from build123d import *

# Parameters (mm, degrees)
EXTRUDE_THIN2_DEPTH     = 165.4
SKETCH11_W              = 166
SKETCH11_H              = 4
BOSS_EXTRUDE3_DEPTH     = 2.6416
CUT_EXTRUDE6_DEPTH      = 270.69086006
CUT_EXTRUDE6_DEPTH_BACK = 270.69086006
SKETCH13_W              = 110.495011338
SKETCH13_H              = 5
CUT_EXTRUDE7_DEPTH      = 273.127102656
SKETCH19_W              = 4
SKETCH19_H              = 155.4
CUT_EXTRUDE9_DEPTH      = 10
SKETCH20_W              = 4
SKETCH20_H              = 155.4
CUT_EXTRUDE10_DEPTH     = 10
SKETCH21_W              = 6
SKETCH21_H              = 86.697
BOSS_EXTRUDE4_DEPTH     = 110
CUT_EXTRUDE11_DEPTH     = 4
SKETCH23_W              = 166
SKETCH23_H              = 4
BOSS_EXTRUDE5_DEPTH     = 2.6416
SKETCH24_W              = 4.14
SKETCH24_H              = 4
BOSS_EXTRUDE6_DEPTH     = 49.64
SKETCH25_W              = 4.14
SKETCH25_H              = 4
BOSS_EXTRUDE7_DEPTH     = 49.64
SKETCH26_W              = 4.14
SKETCH26_H              = 4
BOSS_EXTRUDE8_DEPTH     = 49.64
SKETCH27_W              = 4.14
SKETCH27_H              = 4
BOSS_EXTRUDE9_DEPTH     = 49.64


with BuildPart() as part:
    # Sketch2 → Extrude-Thin2 (new body)
    with BuildSketch(Plane.XY):
        Polygon((0, 120), (0, 0), (186, 0), (186, 120), (176, 120), (176, 10), (10, 10), (10, 120), align=None)
    extrude(amount=EXTRUDE_THIN2_DEPTH)

    # Sketch11 → Boss-Extrude3 (add)
    with BuildSketch(Plane(origin=(0, 10, 0), x_dir=(1, 0, 0), z_dir=(0, 1, 0))):
        with Locations((93, -34.703)):
            Rectangle(SKETCH11_W, SKETCH11_H)
    extrude(amount=BOSS_EXTRUDE3_DEPTH)

    # Sketch13 → Cut-Extrude6 (cut, two sides: drawn at the far end of the back side and taken through both)
    with BuildSketch(Plane(origin=(10, 0, 0), x_dir=(0, 0, -1), z_dir=(1, 0, 0)).offset(-CUT_EXTRUDE6_DEPTH_BACK)):
        with Locations((-103.947505669, 89.551599899)):
            Rectangle(SKETCH13_W, SKETCH13_H)
    extrude(amount=CUT_EXTRUDE6_DEPTH + CUT_EXTRUDE6_DEPTH_BACK, mode=Mode.SUBTRACT)

    # Sketch14 → Cut-Extrude7 (cut, through all)
    with BuildSketch(Plane(origin=(0, 10, 0), x_dir=(1, 0, 0), z_dir=(0, 1, 0))):
        with BuildLine():
            Line((176, -165.4), (10, -165.4))
            ThreePointArc((10, -165.4), (93, -135.4), (176, -165.4))
        make_face()
    extrude(amount=-CUT_EXTRUDE7_DEPTH, mode=Mode.SUBTRACT)

    # Sketch19 → Cut-Extrude9 (cut)
    with BuildSketch(Plane(origin=(0, 120, 0), x_dir=(1, 0, 0), z_dir=(0, 1, 0))):
        with Locations((5, -82.7)):
            Rectangle(SKETCH19_W, SKETCH19_H)
    extrude(amount=-CUT_EXTRUDE9_DEPTH, mode=Mode.SUBTRACT)

    # Sketch20 → Cut-Extrude10 (cut)
    with BuildSketch(Plane(origin=(0, 120, 0), x_dir=(1, 0, 0), z_dir=(0, 1, 0))):
        with Locations((181, -82.7)):
            Rectangle(SKETCH20_W, SKETCH20_H)
    extrude(amount=-CUT_EXTRUDE10_DEPTH, mode=Mode.SUBTRACT)

    # Sketch21 → Boss-Extrude4 (add, through all)
    with BuildSketch(Plane(origin=(0, 10, 0), x_dir=(1, 0, 0), z_dir=(0, 1, 0))):
        with Locations((93, -82.0515)):
            Rectangle(SKETCH21_W, SKETCH21_H)
    extrude(amount=BOSS_EXTRUDE4_DEPTH)

    # Sketch22 → Cut-Extrude11 (cut)
    with BuildSketch(Plane(origin=(0, 10, 0), x_dir=(1, 0, 0), z_dir=(0, 1, 0))):
        Polygon((36, -48.703), (36, -148.583194008), (42, -145.837577441), (42, -48.703), align=None)
        Polygon((144, -145.837577441), (150, -148.583194008), (150, -48.703), (144, -48.703), align=None)
    extrude(amount=-CUT_EXTRUDE11_DEPTH, mode=Mode.SUBTRACT)

    # Sketch23 → Boss-Extrude5 (add)
    with BuildSketch(Plane(origin=(0, 10, 0), x_dir=(1, 0, 0), z_dir=(0, 1, 0))):
        with Locations((93, -27.263)):
            Rectangle(SKETCH23_W, SKETCH23_H)
    extrude(amount=BOSS_EXTRUDE5_DEPTH)

    # Sketch24 → Boss-Extrude6 (add)
    with BuildSketch(Plane(origin=(0, 12.6416, 0), x_dir=(1, 0, 0), z_dir=(0, 1, 0))):
        with Locations((12.07, -27.263)):
            Rectangle(SKETCH24_W, SKETCH24_H)
    extrude(amount=BOSS_EXTRUDE6_DEPTH)

    # Sketch25 → Boss-Extrude7 (add)
    with BuildSketch(Plane(origin=(0, 12.6416, 0), x_dir=(1, 0, 0), z_dir=(0, 1, 0))):
        with Locations((173.93, -27.263)):
            Rectangle(SKETCH25_W, SKETCH25_H)
    extrude(amount=BOSS_EXTRUDE7_DEPTH)

    # Sketch26 → Boss-Extrude8 (add)
    with BuildSketch(Plane(origin=(0, 12.6416, 0), x_dir=(1, 0, 0), z_dir=(0, 1, 0))):
        with Locations((12.07, -34.703)):
            Rectangle(SKETCH26_W, SKETCH26_H)
    extrude(amount=BOSS_EXTRUDE8_DEPTH)

    # Sketch27 → Boss-Extrude9 (add)
    with BuildSketch(Plane(origin=(0, 12.6416, 0), x_dir=(1, 0, 0), z_dir=(0, 1, 0))):
        with Locations((173.93, -34.703)):
            Rectangle(SKETCH27_W, SKETCH27_H)
    extrude(amount=BOSS_EXTRUDE9_DEPTH)


solid = part.part
Check sheet for the modelled part. Datum: model origin and axes. Units: mm. A direction names the side the tool comes from. Give positions to 0.01 mm unless a question says otherwise; leave off trailing zeros. Write each loop counter-clockwise with the first axis right and the second up, starting at its lowest first coordinate (ties: lowest second). Pieces come first, ordered by that corner, then holes. Notation, with made-up numbers: (30, -4) -> (51, -4) arc R23 ccw to (51, 8) -> close; hole circle Ø8 at (-33, 22.25). An arc over 180 degrees is marked (long way). One line per item, written item: value. Start each with the question number.
Item 1: Tool access check on faces 1 (the flat face through (5, 90, 48.7)), 2 (the flat face through (39, 6, 98)), 3 (the flat face through (179, 115, 84)), 4 (the flat face through (93, 11, 25.263)), 5 (the flat face through (181, 87.052, 105)). Record the directions out of +Z, -Z, +X, -X, +Y, -Y that give a thin tool (end or side, any length) a straight path to the whole face; none if there is none.
Item 2: Draft check along Z on faces 6 (the flat face through (76, 10, 86)), 7 (the flat face through (7, 115, 84)), 8 (the flat face through (5, 61, 165.4)). Enter one of: +Z half, -Z half, draft (parallel to the pull), parting line (faces both ways), or undercut.
Item 3: Section check D-D on y = 49. Record the cut outline in (x, z).
Item 4: Section check A-A on y = 75. Record the cut outline in (x, z), then the cut area to 3 significant figures.
Item 5: Material ranges on probe 1 along X at (y, z) = (16.5, 46.5); probe 2 along X at (y, z) = (71.5, 9.5); probe 3 along X at (y, z) = (50, 27), recorded low to high. Write a range as from..to.
Item 6: Section check C-C on x = 147. Record the cut outline in (y, z), then the cut area to 3 significant figures.
Item 7: Section check B-B on z = 10.5. Record the cut outline in (x, y), then the cut area to 3 significant figures.
Item 8: Gauge pin test, flat ends, axial feed: pin 1 (4.5 mm diameter, centred on x = 173.5, z = 34.5, fed in from +Y); pin 2 (3 mm diameter, centred on x = 44, z = 144.5, fed in from +Y); pin 3 (10 mm diameter, centred on x = 115.5, y = 16, fed in from +Z). Record the tip position at first contact, or that the pin passes through.
Results list:
1. face 1: -X
1. face 2: +Z, +Y
1. face 3: +Y
1. face 4: -Z, +Y
1. face 5: +X
2. face 6: draft
2. face 7: undercut
2. face 8: +Z half
3. outline: (0, 0) -> (10, 0) -> (10, 25.26) -> (14.14, 25.26) -> (14.14, 29.26) -> (10, 29.26) -> (10, 32.7) -> (14.14, 32.7) -> (14.14, 36.7) -> (10, 36.7) -> (10, 165.4) -> (0, 165.4) -> close; (90, 38.7) -> (96, 38.7) -> (96, 125.4) -> (90, 125.4) -> close; (171.86, 25.26) -> (176, 25.26) -> (176, 0) -> (186, 0) -> (186, 165.4) -> (176, 165.4) -> (176, 36.7) -> (171.86, 36.7) -> (171.86, 32.7) -> (176, 32.7) -> (176, 29.26) -> (171.86, 29.26) -> close
4. outline: (0, 0) -> (10, 0) -> (10, 165.4) -> (0, 165.4) -> close; (90, 38.7) -> (96, 38.7) -> (96, 125.4) -> (90, 125.4) -> close; (176, 0) -> (186, 0) -> (186, 165.4) -> (176, 165.4) -> close
4. area: 3,830 mm²
5. probe 1: 0..10, 90..96, 176..186
5. probe 2: 0..10, 176..186
5. probe 3: 0..14.14, 171.86..186
6. outline: (0, 0) -> (10, 0) -> (10, 25.26) -> (12.64, 25.26) -> (12.64, 29.26) -> (10, 29.26) -> (10, 32.7) -> (12.64, 32.7) -> (12.64, 36.7) -> (10, 36.7) -> (10, 48.7) -> (6, 48.7) -> (6, 147.16) -> (0, 147.16) -> close
6. area: 1,100 mm²
7. outline: (0, 0) -> (186, 0) -> (186, 120) -> (183, 120) -> (183, 110) -> (179, 110) -> (179, 120) -> (176, 120) -> (176, 10) -> (10, 10) -> (10, 120) -> (7, 120) -> (7, 110) -> (3, 110) -> (3, 120) -> (0, 120) -> close
7. area: 3,980 mm²
8. pin 1: y = 62.28
8. pin 2: y = 10
8. pin 3: z = 36.7
